from build123d import *

# Parameters (mm, degrees)
F0_W     = 129.016124
F0_H     = 66.341627
F0_W_2   = 118.348129
F0_H_2   = 52.339877
F1_DEPTH = 57.658
F3_W     = 64.341373
F3_H     = 31.337252
F4_DEPTH = 139.446
F6_R     = 6.010004
F7_DEPTH = 240.792


with BuildPart() as f1:
    # F0 (on Top) → F1 (new body)
    with BuildSketch(Plane.XY):
        with Locations((2.500314, 0.833438)):
            Rectangle(F0_W, F0_H)
        with Locations((2.500314, 1.500186)):
            Rectangle(F0_W_2, F0_H_2, mode=Mode.SUBTRACT)
    extrude(amount=F1_DEPTH)

    # F3 (on offset) → F4 (cut)
    with BuildSketch(Plane.XZ.offset(68.834)):
        with Locations((0.500061, 42.672002)):
            Rectangle(F3_W, F3_H)
    extrude(amount=-F4_DEPTH, mode=Mode.SUBTRACT)

    # F6 (on offset) → F7 (cut)
    with BuildSketch(Plane.YZ.offset(71.628)):
        with Locations((0, 31.33725)):
            Circle(F6_R)
    extrude(amount=-F7_DEPTH, mode=Mode.SUBTRACT)


solid = f1.part
For this review, take the finished solid that the model builds, in its own axes (mm). A direction names the side the tool comes from. Round coordinates to 2 decimals unless told otherwise and drop trailing zeros. Write each loop counter-clockwise with the first axis right and the second up, starting at its lowest first coordinate (ties: lowest second). Pieces come first, ordered by that corner, then holes. Notation, with made-up numbers: (23.5, 65.5) -> (80.5, 65.5) arc R15 ccw to (80.5, 90.5) -> close; hole circle Ø6 at (86, 26.5). An arc over 180 degrees is marked (long way). Use CSV: the item, a comma, the result in double quotes.
(1) Consider section A-A, the plane z = 51. Give the boundary of the cut face in (x, y).
Computed values:
outline,"(-62.01, -32.34) -> (-31.67, -32.34) -> (-31.67, -24.67) -> (-56.67, -24.67) -> (-56.67, 27.67) -> (-31.67, 27.67) -> (-31.67, 34) -> (-62.01, 34) -> close; (32.67, -32.34) -> (67.01, -32.34) -> (67.01, 34) -> (32.67, 34) -> (32.67, 27.67) -> (61.67, 27.67) -> (61.67, -24.67) -> (32.67, -24.67) -> close"
(2) Clearance check with a flat-ended pin moving along its axis: P1, Ø7, axis at x = 7, y = 31, coming from the +Z side. State where the tip first meets the part, or that it passes through.
Computed values:
P1,"z = 27"
(3) Consider section B-B, the plane y = -16. Give the boundary of the cut face in (x, z).
Computed values:
outline,"(-62.01, 0) -> (-56.67, 0) -> (-56.67, 57.66) -> (-62.01, 57.66) -> close; (61.67, 0) -> (67.01, 0) -> (67.01, 57.66) -> (61.67, 57.66) -> close"
(4) Consider section C-C, the plane x = -8. Give the boundary of the cut face in (y, z).
Computed values:
outline,"(-32.34, 0) -> (-24.67, 0) -> (-24.67, 27) -> (-32.34, 27) -> close; (27.67, 0) -> (34, 0) -> (34, 27) -> (27.67, 27) -> close"
(5) For faces 5 (the face through (2, -24.67, 22)), 6 (the face through (32.671, -29, 42)), 7 (the face through (67.008, 0, 22)), list the 3-axis set-ups (+Z, -Z, +X, -X, +Y, -Y) from which the entire face can be reached by the end or side of a thin tool; tool diameter is ignored.
Computed values:
face 5,"+Z, -Z"
face 6,"+Z, +Y, -Y"
face 7,"+Z, -Z, +X, +Y, -Y"
(6) To check wall thickness, follow L1, parallel to Z at x = 65, y = 0; L2, parallel to Y at x = -8, z = 14.5; L3, parallel to X at y = 15.5, z = 48. State the ranges of each line that lie inside material, in increasing order. Write a range as [from, to].
Computed values:
L1,"[0, 25.33], [37.35, 57.66]"
L2,"[-32.34, -24.67], [27.67, 34]"
L3,"[-62.01, -56.67], [61.67, 67.01]"
(7) Consider section D-D, the plane y = 0. Give the boundary of the cut face in (x, z).
Computed values:
outline,"(-62.01, 0) -> (-56.67, 0) -> (-56.67, 25.33) -> (-62.01, 25.33) -> close; (-62.01, 37.35) -> (-56.67, 37.35) -> (-56.67, 57.66) -> (-62.01, 57.66) -> close; (61.67, 0) -> (67.01, 0) -> (67.01, 25.33) -> (61.67, 25.33) -> close; (61.67, 37.35) -> (67.01, 37.35) -> (67.01, 57.66) -> (61.67, 57.66) -> close"
(8) Draft analysis for pull direction Y (two halves, no side actions). For faces 1 (the face through (-56.674, 7, 28)), 2 (the face through (0, -29, 27.003)), 3 (the face through (2, 27.67, 22)), 4 (the face through (2, -32.337, 22)), state which applies: +Y half, -Y half, draft (parallel to the pull), parting line (faces both ways), or undercut.
Computed values:
face 1,"undercut"
face 2,"draft"
face 3,"undercut"
face 4,"-Y half"
